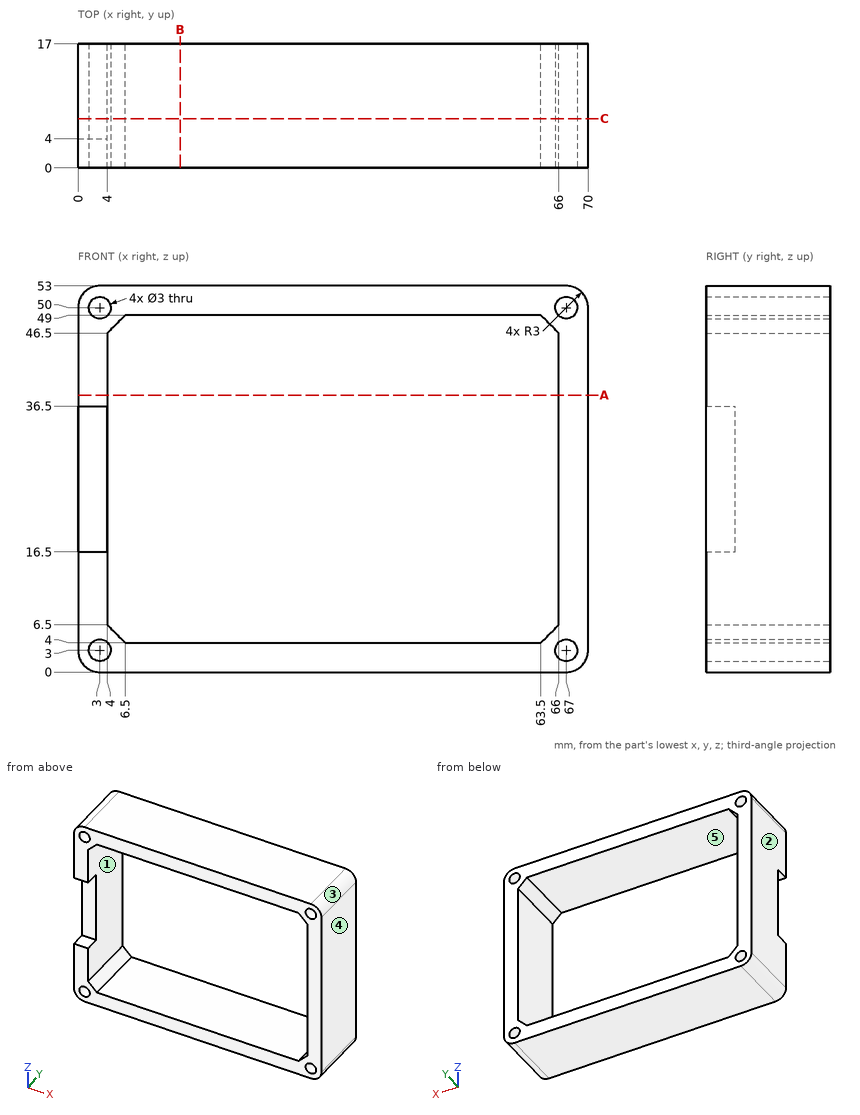
Check sheet for the drawn part. Datum: minimum x, y, z corner. Units: mm. A direction names the side the tool comes from. Round coordinates to 2 decimals unless told otherwise and drop trailing zeros. Order: outer loops, then holes, each group sorted by start corner. A loop starts at its lowest first (then second) coordinate and runs counter-clockwise, first axis right, second up.
(1) Cross-section at C-C, the plane y = 6.75. Enter the section's corners in (x, z).
(2) Go/stop test with flat-tipped pins: P1, Ø2, axis at x = 3, z = 26, coming from the -Y side; P2, Ø2, axis at x = 1.5, y = 3, coming from the -Z side. Record where each tip stops, or that it passes through.
(3) Access from +Z, -Z, +X, -X, +Y, -Y to the whole of each face (thin tool, end or side, straight path). Record for the marked faces 4 and 5.
(4) Cross-section at A-A, the plane z = 38. Enter the section's corners in (x, y), and give its area (3 significant figures).
(5) Cross-section at B-B, the plane x = 14. Enter the section's corners in (y, z).
(6) Scan lines: probe 1 along Z at (x, y) = (3, 5.75); probe 2 along X at (y, z) = (14, 3); probe 3 along X at (y, z) = (10.5, 17). Record each from-to range of solid material in increasing order.
(7) Draft check along X on the marked faces 1, 2 and 3. Enter one of: pulls with the +X half, pulls with the -X half, needs draft (parallel to the pull), parting line crosses it, or undercut.
Check sheet entries:
1. outline: (0, 3) arc R3 ccw to (3, 0) - (67, 0) arc R3 ccw to (70, 3) - (70, 50) arc R3 ccw to (67, 53) - (3, 53) arc R3 ccw to (0, 50) - close; hole circle Ø3 at (3, 3); hole circle Ø3 at (3, 50); hole (4, 6.5) - (6.5, 4) - (63.5, 4) - (66, 6.5) - (66, 46.5) - (63.5, 49) - (6.5, 49) - (4, 46.5) - close; hole circle Ø3 at (67, 3); hole circle Ø3 at (67, 50)
2. P1: stops at y = 4
2. P2: stops at z = 0.04
3. face 4: +Z, -Z, +X, +Y, -Y
3. face 5: +Y, -Y
4. outline: (0, 0) - (4, 0) - (4, 17) - (0, 17) - close; (66, 0) - (70, 0) - (70, 17) - (66, 17) - close
4. area: 136 mm2
5. outline: (0, 0) - (17, 0) - (17, 4) - (0, 4) - close; (0, 49) - (17, 49) - (17, 53) - (0, 53) - close
6. probe 1: z = 0 to 1.5, 4.5 to 48.5, 51.5 to 53
6. probe 2: x = 0 to 1.5, 4.5 to 65.5, 68.5 to 70
6. probe 3: x = 0 to 4, 66 to 70
7. face 1: undercut
7. face 2: pulls with the -X half
7. face 3: pulls with the +X half
